Here's how the part is built. I have some questions about the finished solid (model axes, mm). Face numbers are marked on the shaded views. A direction names the side the tool comes from. Round coordinates to 2 decimals unless told otherwise and drop trailing zeros. Loops run counter-clockwise (first coordinate to the right, second up) from the corner with the lowest first, then second, coordinate; pieces in that order, holes last. Notation, with made-up numbers: (-36, 60) -> (-8, 60) arc R22 cw to (-8, 82) -> close; hole circle Ø10 at (-37.5, -1.5). An arc over 180 degrees is marked (long way). Use one line per item in the form item = value. Start each with the question number.
Item 1: If I drill on L1, parallel to Z at x = -9, y = 11; L2, parallel to X at y = -0.5, z = 12.25; L3, parallel to Y at x = -11.5, z = -0.75, over which ranges is the centre line in solid material (lowest first)? Write a range as [from, to].
Item 2: If we section it at A-A (z = 8.75): Write out the boundary of the cut face in (x, y), then the cut area to 3 significant figures.
Item 3: If we section it at D-D (z = 12): Write out the boundary of the cut face in (x, y).
Item 4: Thinking about a two-plate mould opening in Z: for the marked faces 4, 5, 6 and 7, which applies, released by +Z, released by -Z, zero draft, split by the parting line, or undercut?
Item 5: I'm going to push flat-ended pins straight in: pin 1 Ø2.5 at (y, z) = (19, 13.5) entering from +X; pin 2 Ø2 at (x, z) = (-8.5, 12) entering from +Y; pin 3 Ø2 at (y, z) = (-4, -2) entering from -X. Where does each tip first touch, or does it pass through?
Item 6: If we section it at C-C (y = 0): State how many separate pieces and enclosed holes the cut face has, then the cut area to 3 significant figures.
Item 7: If we section it at B-B (x = 1): Write out the boundary of the cut face in (y, z), then the cut area to 3 significant figures.
Item 8: For the marked faces 1, 2 and 3, which set-ups out of +Z, -Z, +X, -X, +Y, -Y let a thin tool reach every point of the face, with its end or its side?
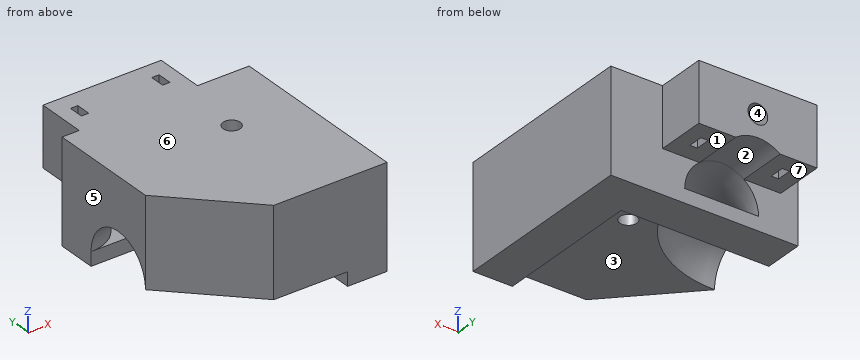
```python
from build123d import *

# Parameters (mm, degrees)
F0_R      = 1.75
F1_DEPTH  = 18
F2_DEPTH  = 2.8
F6_R      = 2
F7_DEPTH  = 10
F8_DEPTH  = 20
F9_W      = 1.5
F9_H      = 3
F10_DEPTH = 25


with BuildPart() as f1:
    # F0 (on Top) → F1 (new body)
    with BuildSketch(Plane.XY):
        Polygon((5.5, -24.5), (5.5, 0), (5.5, 5.5), (0, 5.5), (-24.5, 5.5), (-24.5, -9.5), (-9.5, -24.5), align=None)
        Circle(F0_R, mode=Mode.SUBTRACT)
        Polygon((5.5, 5.5), (5.5, 0), (5.5, -24.5), (13.5, -24.5), (13.5, 0), (13.5, 13.5), (0, 13.5), (-24.5, 13.5), (-24.5, 5.5), (0, 5.5), align=None)
    extrude(amount=F1_DEPTH)

    # F0 (on Top) → F2 (join)
    with BuildSketch(Plane.XY):
        Polygon((5.5, 5.5), (5.5, 0), (5.5, -24.5), (13.5, -24.5), (13.5, 0), (13.5, 13.5), (0, 13.5), (-24.5, 13.5), (-24.5, 5.5), (0, 5.5), align=None)
    extrude(amount=-F2_DEPTH)

    # F5: sweep along a path in F3
    with BuildLine(Plane.XY) as f5_path:
        ThreePointArc((-24.5, -2), (-13.5398448916, 2.5398448916), (-9, 13.5))
    # F4 (on face) → F5 (sweep, cut)
    with BuildSketch(Plane(origin=(-24.5, 0, 0), x_dir=(0, -1, 0), z_dir=(-1, 0, 0))):
        with BuildLine():
            Line((-5.5, 0), (9.5, 0))
            ThreePointArc((9.5, 0), (2, 7.5), (-5.5, 0))
        make_face()
    sweep(path=f5_path.line, mode=Mode.SUBTRACT)

    # F6 (on face) → F7 (join)
    with BuildSketch(Plane(origin=(0, 13.5, 0), x_dir=(-1, 0, 0), z_dir=(0, 1, 0))):
        with BuildLine():
            Line((21, 6), (21, 18))
            Line((21, 18), (-3, 18))
            Line((-3, 18), (-3, 6))
            Line((-3, 6), (4.5, 6))
            ThreePointArc((4.5, 6), (9, 7.5), (13.5, 6))
            Line((13.5, 6), (21, 6))
        make_face()
        with Locations((9, 12)):
            Circle(F6_R, mode=Mode.SUBTRACT)
    extrude(amount=F7_DEPTH)

    # F8 (cut): a face of the model
    f8_faces = [f1.faces().sort_by_distance(p)[0] for p in [
        (-9, 13.5, 12),
    ]]
    extrude(f8_faces, amount=-F8_DEPTH, mode=Mode.SUBTRACT)

    # F9 (on face) → F10 (cut)
    with BuildSketch(Plane(origin=(0, 0, 6), x_dir=(1, 0, 0), z_dir=(0, 0, -1))):
        with Locations((-17.25, -18.5)):
            Rectangle(F9_W, F9_H)
        with Locations((-0.75, -18.5)):
            Rectangle(F9_W, F9_H)
    extrude(amount=-F10_DEPTH, mode=Mode.SUBTRACT)


solid = f1.part
```
Values found:
q1.L1 = [-2.8, 0], [7.5, 10], [14, 18]
q1.L2 = [-24.5, -10.98], [-7.02, -1.68], [1.68, 13.5]
q1.L3 = [5.5, 13.5]
q2.outline = (-24.5, -9.5) -> (-9.5, -24.5) -> (13.5, -24.5) -> (13.5, 13.5) -> (3, 13.5) -> (3, 23.5) -> (-21, 23.5) -> (-21, 13.5) -> (-24.5, 13.5) -> close; hole (-18, 17) -> (-16.5, 17) -> (-16.5, 20) -> (-18, 20) -> close; hole circle Ø3.5 at (0, 0); hole (-1.5, 17) -> (0, 17) -> (0, 20) -> (-1.5, 20) -> close
q2.area = 1,550 mm2
q3.outline = (-24.5, -9.5) -> (-9.5, -24.5) -> (13.5, -24.5) -> (13.5, 13.5) -> (3, 13.5) -> (3, 23.5) -> (-7, 23.5) -> (-7, -6.5) -> (-11, -6.5) -> (-11, 23.5) -> (-21, 23.5) -> (-21, 13.5) -> (-24.5, 13.5) -> close; hole (-18, 17) -> (-16.5, 17) -> (-16.5, 20) -> (-18, 20) -> close; hole circle Ø3.5 at (0, 0); hole (-1.5, 17) -> (0, 17) -> (0, 20) -> (-1.5, 20) -> close
q4.face_4 = undercut
q4.face_5 = zero draft
q4.face_6 = released by +Z
q4.face_7 = released by -Z
q5.pin_1 = 3
q5.pin_2 = -6.5
q5.pin_3 = 5.5
q6.separate_pieces = 2
q6.enclosed_holes = 1
q6.area = 508 mm2
q7.outline = (-24.5, 0) -> (-1.44, 0) -> (-1.44, 18) -> (-24.5, 18) -> close; (1.44, 0) -> (5.5, 0) -> (5.5, -2.8) -> (13.5, -2.8) -> (13.5, 6) -> (23.5, 6) -> (23.5, 18) -> (1.44, 18) -> close
q7.area = 775 mm2
q8.face_1 = -Z, +X, -X, +Y
q8.face_2 = -Z, +Y
q8.face_3 = -Z, -X, -Y
